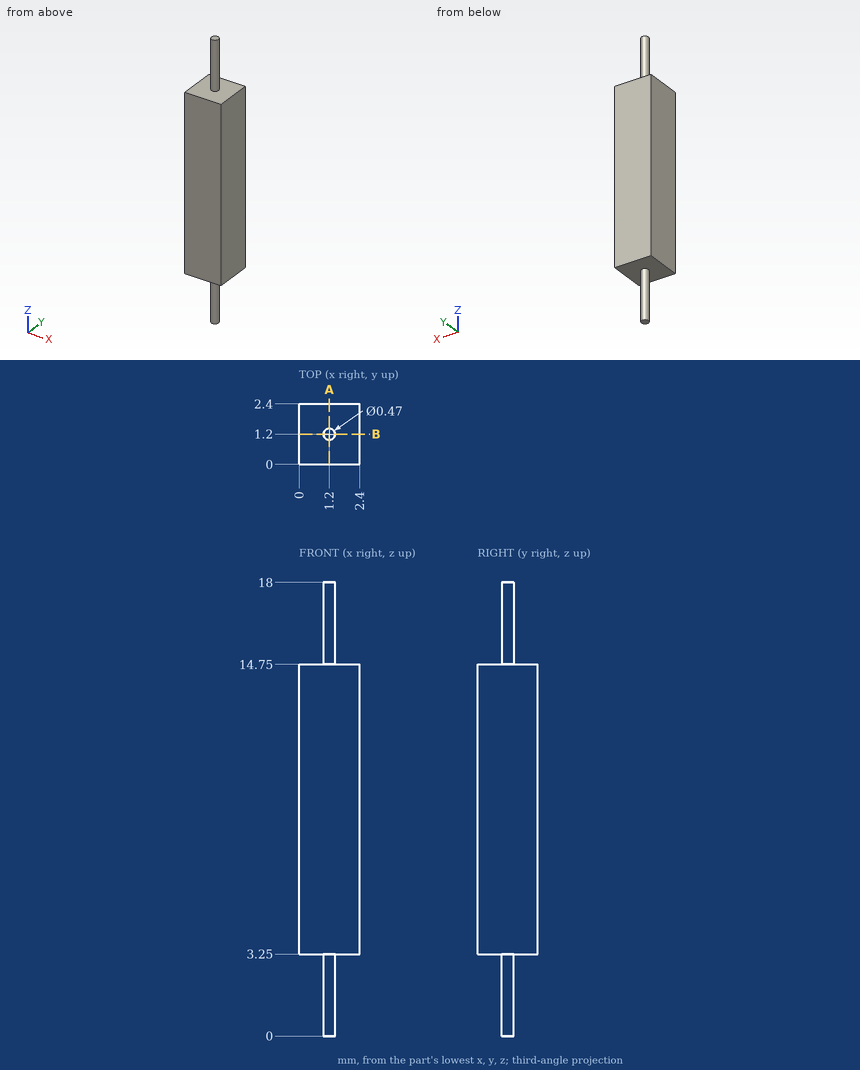
Geometry check sheet. Reference: drawing and pictorial views, mm from the part's lowest x, y, z. Give positions to 0.01 mm unless a question says otherwise; leave off trailing zeros. Loops run counter-clockwise (first coordinate to the right, second up) from the corner with the lowest first, then second, coordinate; pieces in that order, holes last.
1. Go/stop test with a flat-tipped pin: pin 1 Ø1 at (x, y) = (2, 2) entering from -Z. Record where the tip stops, or that it passes through.
2. Thickness scan on line 1 (Z direction, x = 2, y = 0.6); line 2 (X direction, y = 1.25, z = 16.5). Record the ranges inside material, lowest first.
3. Section check A-A, the plane x = 1.2. Enter the section's corners in (y, z) (3 decimals).
Geometry says:
1. pin 1: stops at z = 3.25
2. line 1: z = 3.25 to 14.75
2. line 2: x = 0.97 to 1.43
3. outline: (0, 3.25) - (0.965, 3.25) - (0.965, 0) - (1.435, 0) - (1.435, 3.25) - (2.4, 3.25) - (2.4, 14.75) - (1.435, 14.75) - (1.435, 18) - (0.965, 18) - (0.965, 14.75) - (0, 14.75) - close
